Read the model definition and answer for the solid it produces. Units are mm, in the model's axes. Face numbers are marked on the shaded views. A direction names the side the tool comes from. Give positions to 0.01 mm unless a question says otherwise; leave off trailing zeros. Order: outer loops, then holes, each group sorted by start corner. A loop starts at its lowest first (then second) coordinate and runs counter-clockwise, first axis right, second up. Notation, with made-up numbers: (48, 38) - (71, 38) arc R17 ccw to (71, 46) - close; hole circle Ø6 at (23.25, -30.5). An arc over 180 degrees is marked (long way). Write each question's results on one line, items separated by ' | '. Start each with the question number.
Q1. Find the intervals of material crossed by line 1 along Z through (x, y) = (5, -7); line 2 along Y through (x, z) = (0, 17) (3 decimals); line 3 along Z through (x, y) = (10, 7.25), in increasing order. Write a range as from..to.
Q2. Flat-ended cylindrical pins translate along their axes: P1, Ø1.5, axis at x = -3.5, z = 29, coming from the +Y side; P2, Ø2, axis at x = 2, y = -3.5, coming from the +Z side; P3, Ø12, axis at x = 9.5, z = 46, coming from the -Y side. Find the tip coordinate at first contact, or state that the pin passes through.
Q3. Find section A-A on x = 0. Give the vertices of the cut face in (y, z) (1 decimal), and give its area (3 significant figures).
Q4. Find section D-D on x = -9. Give the vertices of the cut face in (y, z).
Q5. Find section C-C on z = 22. Give the vertices of the cut face in (x, y) (3 decimals).
Q6. A tool of negligible diameter and unlimited length cuts with its end or side. For the marked faces 1, 2 and 3, from which of +Z, -Z, +X, -X, +Y, -Y can it reach the whole face along a straight path? Write none if from no direction.
from build123d import *

# Parameters (mm, degrees)
SKETCH1_R           = 12.7
BOSS_EXTRUDE1_DEPTH = 50.8
SKETCH2_R           = 3.4925
BOSS_EXTRUDE2_DEPTH = 2.54
SKETCH3_R           = 1.9685
BOSS_EXTRUDE3_DEPTH = 9.525
SKETCH4_OUTSIDE_W   = 41.88
SKETCH4_OUTSIDE_H   = 41.88
SKETCH4_OUTSIDE_R   = 12.065
CUT_EXTRUDE1_DEPTH  = 30.48


with BuildPart() as part:
    # Sketch1 → Boss-Extrude1 (new body)
    with BuildSketch(Plane.XY):
        Circle(SKETCH1_R)
    extrude(amount=BOSS_EXTRUDE1_DEPTH)

    # Sketch2 → Boss-Extrude2 (add)
    with BuildSketch(Plane.XY.offset(50.8)):
        Circle(SKETCH2_R)
    extrude(amount=BOSS_EXTRUDE2_DEPTH)

    # Sketch3 → Boss-Extrude3 (add)
    with BuildSketch(Plane.XY.offset(53.34)):
        Circle(SKETCH3_R)
    extrude(amount=BOSS_EXTRUDE3_DEPTH)

    # Sketch4 outside → Cut-Extrude1 (cut)
    with BuildSketch(Plane(origin=(0, 0, 0), x_dir=(-1, 0, 0), z_dir=(0, 0, -1))):
        Rectangle(SKETCH4_OUTSIDE_W, SKETCH4_OUTSIDE_H)
        Circle(SKETCH4_OUTSIDE_R, mode=Mode.SUBTRACT)
    extrude(amount=-CUT_EXTRUDE1_DEPTH, mode=Mode.SUBTRACT)


solid = part.part
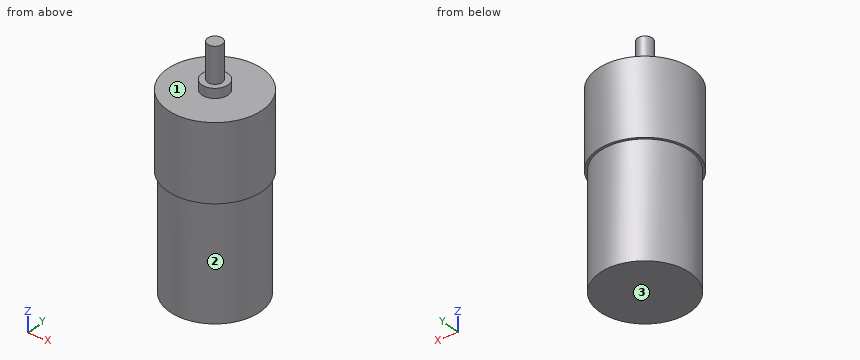
Working result:
1) line 1: 0..50.8 | line 2: -12.065..12.065 | line 3: 30.48..50.8
2) P1: y = 11.75 | P2: z = 53.34 | P3: y = -12.21
3) outline: (-12.7, 30.5) - (-12.1, 30.5) - (-12.1, 0) - (12.1, 0) - (12.1, 30.5) - (12.7, 30.5) - (12.7, 50.8) - (3.5, 50.8) - (3.5, 53.3) - (2, 53.3) - (2, 62.9) - (-2, 62.9) - (-2, 53.3) - (-3.5, 53.3) - (-3.5, 50.8) - (-12.7, 50.8) - close | area: 1,310 mm²
4) outline: (-8.96, 30.48) - (-8.04, 30.48) - (-8.04, 0) - (8.04, 0) - (8.04, 30.48) - (8.96, 30.48) - (8.96, 50.8) - (-8.96, 50.8) - close
5) outline: circle Ø24.13 at (0, 0)
6) face 1: +Z | face 2: -Z | face 3: -Z, +X, -X, +Y, -Y
